Read the model definition and answer for the solid it produces. Units are mm, in the model's axes. A direction names the side the tool comes from. Coordinates: 2 decimals unless noted, no trailing zeros. Order: outer loops, then holes, each group sorted by start corner. A loop starts at its lowest first (then second) coordinate and runs counter-clockwise, first axis right, second up. Notation, with made-up numbers: (75.5, 89.5) - (127.5, 89.5) arc R28 ccw to (127.5, 128.5) - close; hole circle Ø7 at (26.5, 31.5). An arc over 180 degrees is marked (long way). Use one line per item in the form item = value.
```python
from build123d import *

# Parameters (mm, degrees)
F1_DEPTH = 1.5
F2_R     = 2
F3_R     = 1


with BuildPart() as f1:
    # F0 (on Top) → F1 (new body, symmetric)
    with BuildSketch(Plane.XY):
        Polygon((4, 12), (0, 12), (0, 10), (2, 10), (2, -10), (0, -10), (0, -12), (4, -12), align=None)
    extrude(amount=F1_DEPTH, both=True)

    # F2
    f2_edges = [f1.edges().sort_by_distance(p)[0] for p in [
        (4, -12, 0),
        (4, 12, 0),
    ]]
    fillet(f2_edges, radius=F2_R)

    # F3
    f3_edges = [f1.edges().sort_by_distance(p)[0] for p in [
        (2, 10, 0),
        (2, -10, 0),
    ]]
    fillet(f3_edges, radius=F3_R)


solid = f1.part
```
(1) Section B-B, the plane z = 0.35 is taken. Write down the section's boundary in (x, y).
Answer list:
outline = (0, -12) - (2, -12) arc R2 ccw to (4, -10) - (4, 10) arc R2 ccw to (2, 12) - (0, 12) - (0, 10) - (1, 10) arc R1 cw to (2, 9) - (2, -9) arc R1 cw to (1, -10) - (0, -10) - close
(2) Section C-C, the plane y = 4 is taken. Write down the section's boundary in (x, z).
Answer list:
outline = (2, -1.5) - (4, -1.5) - (4, 1.5) - (2, 1.5) - close
(3) The mould has two halves that part along Y. Classify faces 1 (the flat face through (0.5, -10, 0)), 2 (the flat face through (4, 0, 0)), 3 (the flat face through (1, 12, 0)), 4 (the cylindrical face through (1.715, -9.699, 0.021)): +Y half, -Y half, draft (parallel to the pull), parting line (faces both ways), or undercut.
Answer list:
face_1 = undercut
face_2 = draft
face_3 = +Y half
face_4 = undercut
(4) Given pin 1 Ø1.5 at (y, z) = (3.5, -0.5) entering from -X, flat-ended and moving along its own axis, determine where the tip first touches the part or whether it passes through.
Answer list:
pin_1 = 2
(5) Section A-A, the plane x = 0.5 is taken. Write down the section's boundary in (y, z), then the cut area to 3 significant figures.
Answer list:
outline = (-12, -1.5) - (-10, -1.5) - (-10, 1.5) - (-12, 1.5) - close; (10, -1.5) - (12, -1.5) - (12, 1.5) - (10, 1.5) - close
area = 12.0 mm2
(6) Straight lines are drawn through the part: L1, parallel to Y at x = 1.1, z = -0.1; L2, parallel to X at y = -6.75, z = -1.2; L3, parallel to Y at x = 1.4, z = 0.7. For each, find the intervals that lie inside material, in ascending order.
Answer list:
L1 = -12 to -9.99, 9.99 to 12
L2 = 2 to 4
L3 = -12 to -9.92, 9.92 to 12
(7) Section D-D, the plane x = 1.4 is taken. Write down the section's boundary in (y, z).
Answer list:
outline = (-12, -1.5) - (-9.92, -1.5) - (-9.92, 1.5) - (-12, 1.5) - close; (9.92, -1.5) - (12, -1.5) - (12, 1.5) - (9.92, 1.5) - close
(8) Which of the six approach directions +Z, -Z, +X, -X, +Y, -Y give full straight-line access (tool end or side, diameter ignored) to faces 5 (the flat face through (2, 0, 0)), 6 (the flat face through (1, -12, 0))?
Answer list:
face_5 = +Z, -Z, -X
face_6 = +Z, -Z, +X, -X, -Y
